```python
from build123d import *

# Parameters (mm, degrees)
F1_DEPTH    = 6.35
F2_T1_DEPTH = 23.4696
F2_T3_DEPTH = 117.8964839186
F2_T5_DEPTH = 23.4799160814
F2_T7_DEPTH = 117.9413513149
F2_T9_DEPTH = 23.4350486851
F3_R        = 4.318
F5_DEPTH    = 101.6


# Not quite as in the source:
# - a fillet or chamfer that OpenCascade refuses, or shapes differently, is made with other operations: its cross-section is extruded or revolved along the edge and cut away or added


with BuildPart() as f1:
    # F0 (on Front) → F1 (new body)
    with BuildSketch(Plane.XZ):
        Polygon((69.85, -9.525), (69.85, 9.525), (62.8904, 9.525), (62.8904, 4.7625), (50.6984, 4.7625), (50.6984, 9.525), (-50.6880839186, 9.525), (-50.6880839186, 4.7625), (-62.8800839186, 4.7625), (-62.8800839186, 9.525), (-69.85, 9.525), (-69.85, -9.525), (-62.9249513149, -9.525), (-62.9249513149, -4.7625), (-50.7329513149, -4.7625), (-50.7329513149, -9.525), (50.6984, -9.525), (50.6984, -4.7625), (62.8904, -4.7625), (62.8904, -9.525), align=None)
    extrude(amount=F1_DEPTH)

    # F2: fillet of radius 3.302 on 10 edges, made by hand

    # F2_s2 → F2_t1 (cut)
    with BuildSketch(Plane.YZ.offset(54.6354)):
        with BuildLine():
            ThreePointArc((-3.302, 9.525), (-0.9671334085, 8.5578665915), (0, 6.223))
            Line((0, 6.223), (0, 9.525))
            Line((0, 9.525), (-3.302, 9.525))
        make_face()
        with BuildLine():
            ThreePointArc((-3.048, 9.525), (-5.3828665915, 8.5578665915), (-6.35, 6.223))
            Line((-6.35, 6.223), (-6.35, 9.525))
            Line((-6.35, 9.525), (-3.048, 9.525))
        make_face()
        with BuildLine():
            ThreePointArc((-3.302, -9.525), (-0.9671334085, -8.5578665915), (0, -6.223))
            Line((0, -6.223), (0, -9.525))
            Line((0, -9.525), (-3.302, -9.525))
        make_face()
        with BuildLine():
            ThreePointArc((-3.048, -9.525), (-5.3828665915, -8.5578665915), (-6.35, -6.223))
            Line((-6.35, -6.223), (-6.35, -9.525))
            Line((-6.35, -9.525), (-3.048, -9.525))
        make_face()
    extrude(amount=F2_T1_DEPTH, mode=Mode.SUBTRACT)

    # F2_s4 → F2_t3 (cut)
    with BuildSketch(Plane.YZ.offset(-58.9430839186)):
        with BuildLine():
            ThreePointArc((-3.302, 9.525), (-0.9671334085, 8.5578665915), (0, 6.223))
            Line((0, 6.223), (0, 9.525))
            Line((0, 9.525), (-3.302, 9.525))
        make_face()
    extrude(amount=F2_T3_DEPTH, mode=Mode.SUBTRACT)

    # F2_s6 → F2_t5 (cut)
    with BuildSketch(Plane.YZ.offset(-78.105)):
        with BuildLine():
            ThreePointArc((-3.302, 9.525), (-0.9671334085, 8.5578665915), (0, 6.223))
            Line((0, 6.223), (0, 9.525))
            Line((0, 9.525), (-3.302, 9.525))
        make_face()
        with BuildLine():
            ThreePointArc((-3.048, 9.525), (-5.3828665915, 8.5578665915), (-6.35, 6.223))
            Line((-6.35, 6.223), (-6.35, 9.525))
            Line((-6.35, 9.525), (-3.048, 9.525))
        make_face()
    extrude(amount=F2_T5_DEPTH, mode=Mode.SUBTRACT)

    # F2_s8 → F2_t7 (cut)
    with BuildSketch(Plane.YZ.offset(-58.9879513149)):
        with BuildLine():
            ThreePointArc((-3.302, -9.525), (-0.9671334085, -8.5578665915), (0, -6.223))
            Line((0, -6.223), (0, -9.525))
            Line((0, -9.525), (-3.302, -9.525))
        make_face()
    extrude(amount=F2_T7_DEPTH, mode=Mode.SUBTRACT)

    # F2_s10 → F2_t9 (cut)
    with BuildSketch(Plane.YZ.offset(-78.105)):
        with BuildLine():
            ThreePointArc((-3.302, -9.525), (-0.9671334085, -8.5578665915), (0, -6.223))
            Line((0, -6.223), (0, -9.525))
            Line((0, -9.525), (-3.302, -9.525))
        make_face()
        with BuildLine():
            ThreePointArc((-3.048, -9.525), (-5.3828665915, -8.5578665915), (-6.35, -6.223))
            Line((-6.35, -6.223), (-6.35, -9.525))
            Line((-6.35, -9.525), (-3.048, -9.525))
        make_face()
    extrude(amount=F2_T9_DEPTH, mode=Mode.SUBTRACT)

    # F3
    f3_edges = [f1.edges().sort_by_distance(p)[0] for p in [
        (-56.784084, 0, 4.7625),
        (-56.828951, 0, -4.7625),
        (56.7944, 0, -4.7625),
        (56.7944, 0, 4.7625),
    ]]
    fillet(f3_edges, radius=F3_R)

    # F4 (on face) → F5 (join)
    with BuildSketch(Plane.YZ.offset(50.6984)):
        with BuildLine():
            Line((-6.35, 4.7625), (-6.35, 9.525))
            ThreePointArc((-6.35, 9.525), (-11.2043924939, 0.0067562208), (-6.35, -9.5114875585))
            Line((-6.35, -9.5114875585), (-6.35, -4.8156534322))
            Line((-6.35, -4.8156534322), (-6.35, 4.7625))
        make_face()
    extrude(amount=-F5_DEPTH)


solid = f1.part
```
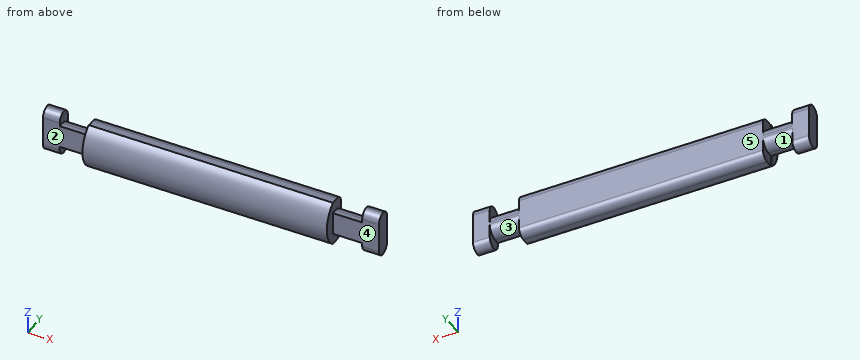
Here's how the part is built. I have some questions about the finished solid (model axes, mm). Face numbers are marked on the shaded views. A direction names the side the tool comes from. Round coordinates to 2 decimals unless told otherwise and drop trailing zeros. Loops run counter-clockwise (first coordinate to the right, second up) from the corner with the lowest first, then second, coordinate; pieces in that order, holes last. Notation, with made-up numbers: (13, -31.75) -> (42, -31.75) arc R5 cw to (42, -22.75) -> close; hole circle Ø4 at (25, 46). An arc over 180 degrees is marked (long way). Answer as CSV lines item,"result".
1. If we section it at C-C on z = 2.75: Please give me the cut outline in (x, y), plus the area to 3 significant figures.
Final values:
outline,"(-69.85, -6.35) -> (-50.9, -6.35) -> (-50.9, -10.88) -> (50.7, -10.88) -> (50.7, -6.35) -> (69.85, -6.35) -> (69.85, 0) -> (62.89, 0) -> (62.89, -0.67) -> (50.7, -0.67) -> (50.7, 0) -> (-50.69, 0) -> (-50.69, -0.67) -> (-62.88, -0.67) -> (-62.88, 0) -> (-69.85, 0) -> close"
area,"1,330 mm^2"
2. If we section it at D-D on x = 60: Please give me the cut outline in (y, z), plus the area to 3 significant figures.
Final values:
outline,"(-6.35, -4.76) -> (-4.32, -4.76) arc R4.32 ccw to (0, -0.44) -> (0, 0.44) arc R4.32 ccw to (-4.32, 4.76) -> (-6.35, 4.76) -> close"
area,"52.5 mm^2"
3. If we section it at A-A on x = 27: Please give me the cut outline in (y, z) (3 decimals), plus the area to 3 significant figures.
Final values:
outline,"(-6.35, -9.525) -> (-3.302, -9.525) arc R3.302 ccw to (0, -6.223) -> (0, 6.223) arc R3.302 ccw to (-3.302, 9.525) -> (-6.35, 9.525) arc R11.759 ccw to (-6.35, -9.511) -> close"
area,"181 mm^2"
4. If we section it at B-B on y = -2: Please give me the cut outline in (x, z), plus the area to 3 significant figures.
Final values:
outline,"(-69.85, -9.26) -> (-62.92, -9.26) -> (-62.92, -4.09) -> (-50.73, -4.09) -> (-50.73, -9.26) -> (50.7, -9.26) -> (50.7, -4.09) -> (62.89, -4.09) -> (62.89, -9.26) -> (69.85, -9.26) -> (69.85, 9.26) -> (62.89, 9.26) -> (62.89, 4.09) -> (50.7, 4.09) -> (50.7, 9.26) -> (-50.69, 9.26) -> (-50.69, 4.09) -> (-62.88, 4.09) -> (-62.88, 9.26) -> (-69.85, 9.26) -> close"
area,"2,330 mm^2"
5. For pin 1 (1.6 mm diameter, centred on x = 55.5, y = -5, fed in from -Z); pin 2 (3 mm diameter, centred on y = -8, z = 2.5, fed in from -X); pin 3 (2 mm diameter, centred on x = 57, y = -5.5, fed in from +Z), each with a flat end and sliding along its axis, tell me the tip position at first contact or that it passes through.
Final values:
pin 1,"stops at z = -4.76"
pin 2,"stops at x = -50.9"
pin 3,"stops at z = 4.76"
6. Thinking about a two-plate mould opening in X: for the marked faces 1 and 2, which applies, released by +X, released by -X, zero draft, split by the parting line, or undercut?
Final values:
face 1,"undercut"
face 2,"zero draft"
7. If I drill on L1, parallel to X at y = -0.75, z = 5; L2, parallel to Z at x = -47, y = -3; L3, parallel to Y at x = -1, z = 0.5, over which ranges is the centre line in solid material (lowest first)?
Final values:
L1,"x = -69.85 to -62.88, -50.69 to 50.7, 62.89 to 69.85"
L2,"z = -9.51 to 9.51"
L3,"y = -11.19 to 0"
8. Which directions (+Z, -Z, +X, -X, +Y, -Y) give clear straight access to the entire face, cutting with the end or side of a thin tool? Please do the marked faces 3, 4 and 5.
Final values:
face 3,"-Z, +Y"
face 4,"+Z, -Z, +X, -Y"
face 5,"+Z, -Z, +X, -X, +Y"
